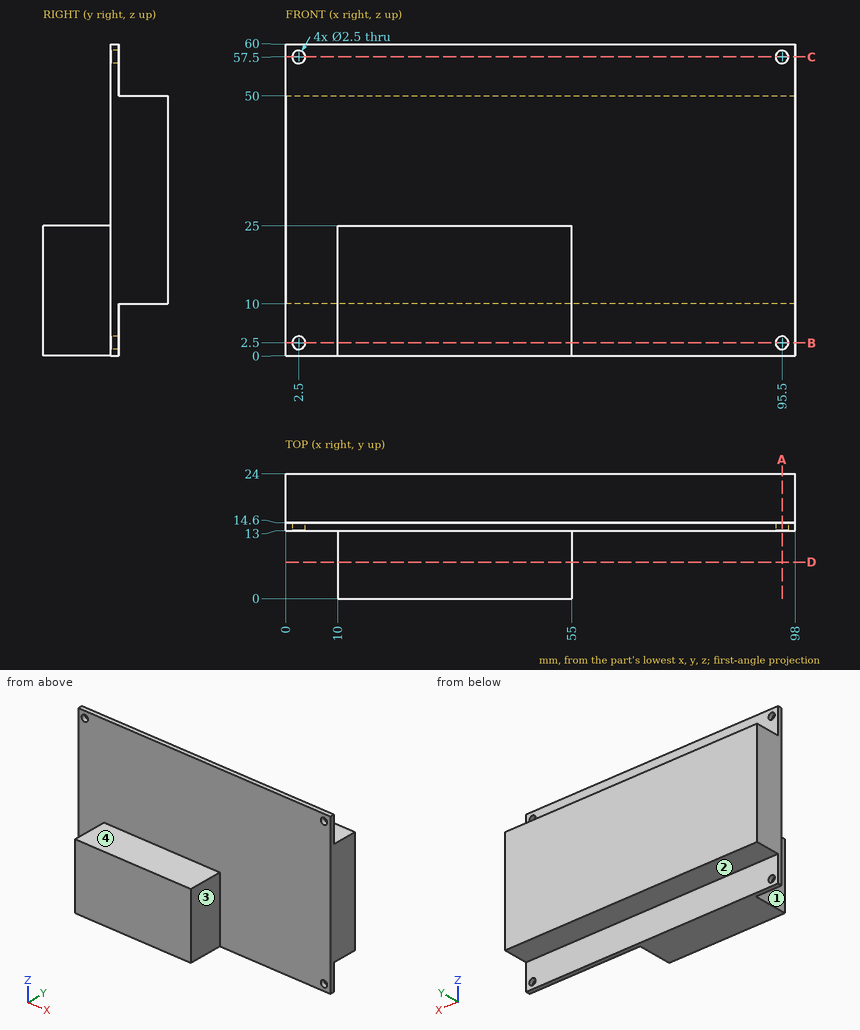
Job drawing, mm, ordinate dimensions from the low corner. One solid piece. A direction names the side the tool comes from. Coordinates: 2 decimals unless noted, no trailing zeros. Write each loop counter-clockwise with the first axis right and the second up, starting at its lowest first coordinate (ties: lowest second). Pieces come first, ordered by that corner, then holes.
Item 1: Pin check, flat tips, straight feed: pin 1 (3 mm diameter, centred on y = 12.5, z = 35.5, fed in from -X); pin 2 (10.5 mm diameter, centred on y = 6, z = 15.5, fed in from +X); pin 3 (4 mm diameter, centred on x = 95.5, z = 2.5, fed in from +Y); pin 4 (6.5 mm diameter, centred on x = 31, y = 5.5, fed in from +Z). Stop position of each tip, or through.
Item 2: Slice it at C-C (z = 57.5). Write the cut outline in (x, y).
Item 3: Slice it at D-D (y = 7). Write the cut outline in (x, z), and give its area (4 significant figures).
Item 4: Slice it at A-A (x = 95.5). Write the cut outline in (y, z), and give its area (3 significant figures).
Item 5: Probe line 1 (X direction, y = 14.05, z = 57.5); line 2 (Z direction, x = 95.5, y = 13.4); line 3 (Z direction, x = 72, y = 17.75). List the from-to ranges inside material, lowest first.
Item 6: Slice it at B-B (z = 2.5). Write the cut outline in (x, y).
Item 7: Which spindle directions (+Z, -Z, +X, -X, +Y, -Y) get a long thin tool onto all of the face, cutting with end or side? Do the marked faces 1, 2, 3 and 4. Say none if no direction does.
Results found:
1. pin 1: stops at x = 0
1. pin 2: stops at x = 55
1. pin 3: stops at y = 14.6
1. pin 4: stops at z = 25
2. outline: (0, 13) - (1.25, 13) - (1.25, 14.6) - (0, 14.6) - close; (3.75, 13) - (94.25, 13) - (94.25, 14.6) - (3.75, 14.6) - close; (96.75, 13) - (98, 13) - (98, 14.6) - (96.75, 14.6) - close
3. outline: (10, 0) - (55, 0) - (55, 25) - (10, 25) - close
3. area: 1,125 mm2
4. outline: (13, 0) - (14.6, 0) - (14.6, 1.25) - (13, 1.25) - close; (13, 3.75) - (14.6, 3.75) - (14.6, 10) - (24, 10) - (24, 50) - (14.6, 50) - (14.6, 56.25) - (13, 56.25) - close; (13, 58.75) - (14.6, 58.75) - (14.6, 60) - (13, 60) - close
4. area: 464 mm2
5. line 1: x = 0 to 1.25, 3.75 to 94.25, 96.75 to 98
5. line 2: z = 0 to 1.25, 3.75 to 56.25, 58.75 to 60
5. line 3: z = 10 to 50
6. outline: (0, 13) - (1.25, 13) - (1.25, 14.6) - (0, 14.6) - close; (3.75, 13) - (10, 13) - (10, 0) - (55, 0) - (55, 13) - (94.25, 13) - (94.25, 14.6) - (3.75, 14.6) - close; (96.75, 13) - (98, 13) - (98, 14.6) - (96.75, 14.6) - close
7. face 1: +Z, -Z, -X, -Y
7. face 2: -Z, +X, -X, +Y
7. face 3: +Z, -Z, +X, -Y
7. face 4: +Z, +X, -X, -Y
